Work out the finished part from the listing and answer in its coordinate system (mm). A direction names the side the tool comes from. Coordinates: 2 decimals unless noted, no trailing zeros. Order: outer loops, then holes, each group sorted by start corner. A loop starts at its lowest first (then second) coordinate and runs counter-clockwise, first axis right, second up. Notation, with made-up numbers: M 73.5,-22.5 L 112.5,-22.5 A12 cw 112.5,-4.5 Z; hole C -19.75,88 d10. An arc over 180 degrees is marked long. Use a Markdown table: item, result.
from build123d import *

# Parameters (mm, degrees)
SWEEP1_START              = -7.5
SWEEP1_DEPTH              = 15
SKETCH4_W                 = 19
SKETCH4_H                 = 5
BOSS_EXTRUDE1_DEPTH       = 10
M3X0_5_TAPPED_HOLE1_D     = 2.5
M3X0_5_TAPPED_HOLE1_DEPTH = 7.5
M3X0_5_TAPPED_HOLE1_TIP   = 0.751075774


with BuildPart() as part:
    # Sketch1 → Revolve1 (revolve)
    with BuildSketch(Plane.XY, mode=Mode.PRIVATE) as revolve1_sk:
        Polygon((0, 0), (-10, 0), (-18, 11), (-18, 68.1), (-16, 68.1), (-16, 96.6), (-10, 96.6), (-10, 100.3), (-3, 100.3), (-3, 115.8), (0, 115.8), align=None)
    revolve(revolve1_sk.sketch.rotate(Axis((0, 115.8, 0), (0, -1, 0)), 270), axis=Axis((0, 115.8, 0), (0, -1, 0)))

    # Sweep1: read off the stored shape, not the designer's step
    # Sweep1 outline → Sweep1 (add)
    with BuildSketch(Plane.XY.offset(SWEEP1_START)):
        with BuildLine():
            add(Edge.make_bspline(
                [(-15.28930073, 9.665917189), (-15.155241069, 9.50042506), (-15.020974619, 9.335100438), (-14.781588664, 9.041143621), (-14.67655559, 8.912441119), (-14.571379426, 8.783855646)],
                knots=[17.713260558, 17.713260558, 17.713260558, 17.713260558, 18.352193294, 18.352193294, 18.850555217, 18.850555217, 18.850555217, 18.850555217], degree=3))
            add(Edge.make_bspline(
                [(-15.28930073, 9.665917189), (-22.240343975, 8.202614741), (-29.318460029, 5.946043988), (-48.487680613, 1.623066579), (-60.300160331, 0.950060594), (-70.622683773, 9.904196742)],
                knots=[0.213963068, 0.213963068, 0.213963068, 0.213963068, 0.5, 0.5, 1, 1, 1, 1], degree=3))
            Line((-70.622683773, 9.904196742), (-71.211326259, 9.095803258))
            add(Edge.make_bspline(
                [(-14.571379426, 8.783855646), (-21.586501057, 7.343246642), (-28.814104178, 5.043485332), (-48.284336953, 0.638583113), (-60.500298128, -0.149792653), (-71.211326259, 9.095803258)],
                knots=[0.207983451, 0.207983451, 0.207983451, 0.207983451, 0.5, 0.5, 1, 1, 1, 1], degree=3))
        make_face()
    extrude(amount=SWEEP1_DEPTH)

    # Sketch4 → Boss-Extrude1 (add)
    with BuildSketch(Plane(origin=(-50.864884567, 37.037943446, 0), x_dir=(0, 0, 1), z_dir=(-0.8083934830959073, 0.5886424861391397, 0))):
        with Locations((0, -34.065024053)):
            Rectangle(SKETCH4_W, SKETCH4_H)
    extrude(amount=BOSS_EXTRUDE1_DEPTH)

    # M3x0.5 Tapped Hole1
    with Locations(Plane(origin=(0, 96.6, 0), x_dir=(1, 0, 0), z_dir=(0, 1, 0))):
        with Locations((9.192388155, 9.192388155), (9.192388155, -9.192388155), (-9.192388155, -9.192388155), (-9.192388155, 9.192388155)):
            Hole(M3X0_5_TAPPED_HOLE1_D / 2, depth=M3X0_5_TAPPED_HOLE1_DEPTH)
            with Locations((0, 0, -(M3X0_5_TAPPED_HOLE1_DEPTH + M3X0_5_TAPPED_HOLE1_TIP / 2))):  # 118° drill point
                Cone(0, M3X0_5_TAPPED_HOLE1_D / 2, M3X0_5_TAPPED_HOLE1_TIP, mode=Mode.SUBTRACT)


solid = part.part
(1) Which of the six approach directions +Z, -Z, +X, -X, +Y, -Y give full straight-line access (tool end or side, diameter ignored) to faces 5 (the flat face through (-73.4, 14.4, -0.1)), 6 (the cylindrical face through (-0.9, 108.16, 2.86)), 7 (the flat face through (-75, 12, 9.5)), 8 (the flat face through (-75, 12, -9.5)), 9 (the flat face through (-76.4, 10.4, -0.1))?
Conclusion:
| item | result |
|---|---|
| face 5 | +Z, -Z, +Y |
| face 6 | +Y |
| face 7 | +Z, -X, +Y, -Y |
| face 8 | -Z, -X, +Y, -Y |
| face 9 | +Z, -Z, -X, -Y |
(2) A cutting plane is placed at C-C (y = 66.5). Determine the outline of the cut face in (x, z), then the cut area to 3 significant figures.
Conclusion:
| item | result |
|---|---|
| outline | C 0,0 d36 |
| area | 1,020 mm2 |
(3) Straight lines are drawn through the part: L1, parallel to Y at x = -1, z = -9; L2, parallel to Y at x = -50, z = 4; L3, parallel to Z at x = -74, y = 12.5. For each, find the intervals that lie inside material, in ascending order.
Conclusion:
| item | result |
|---|---|
| L1 | 0 to 100.3 |
| L2 | 1.55 to 2.55 |
| L3 | -9.5 to 9.5 |
(4) Determine the mould class of faces 1 (the cylindrical face through (-5.407, 39.95, 17.169)), 2 (the cylindrical face through (10.11, 92.8, -10.04)), 3 (the flat face through (0, 0, 0)), 4 (the conical face through (-8.99, 88.48, 9.28)) for opening direction Z: pulls with the +Z half, pulls with the -Z half, needs draft (parallel to the pull), parting line crosses it, or undercut.
Conclusion:
| item | result |
|---|---|
| face 1 | parting line crosses it |
| face 2 | undercut |
| face 3 | needs draft |
| face 4 | undercut |
(5) A cutting plane is placed at A-A (x = 0). Determine the outline of the cut face in (y, z), then the cut area to 3 significant figures.
Conclusion:
| item | result |
|---|---|
| outline | M 0,-10 L 11,-18 L 68.1,-18 L 68.1,-16 L 96.6,-16 L 96.6,-10 L 100.3,-10 L 100.3,-3 L 115.8,-3 L 115.8,3 L 100.3,3 L 100.3,10 L 96.6,10 L 96.6,16 L 68.1,16 L 68.1,18 L 11,18 L 0,10 Z |
| area | 3,440 mm2 |
(6) Given P1, Ø6.5, axis at x = -34.5, y = 7.5, coming from the -Z side; P2, Ø5, axis at y = 73, z = 14, coming from the +X side; P3, Ø16, axis at x = -5, z = -2, coming from the +Y side; P4, Ø1, axis at y = 44, z = -1, coming from the -X side, each flat-ended and moving along its own axis, determine where each tip first touches the part or whether it passes through.
Conclusion:
| item | result |
|---|---|
| P1 | z = -7.5 |
| P2 | x = 11.12 |
| P3 | y = 115.8 |
| P4 | x = -17.99 |
(7) A cutting plane is placed at B-B (y = 98.5). Determine the outline of the cut face in (x, z), then the cut area to 3 significant figures.
Conclusion:
| item | result |
|---|---|
| outline | C 0,0 d20 |
| area | 314 mm2 |
